Design review of the part built by this model. Coordinates are the model's own, in mm. Face numbers are marked on the shaded views. A direction names the side the tool comes from. Give positions to 0.01 mm unless a question says otherwise; leave off trailing zeros. Write each loop counter-clockwise with the first axis right and the second up, starting at its lowest first coordinate (ties: lowest second). Pieces come first, ordered by that corner, then holes. Notation, with made-up numbers: (48.5, 23.5) -> (81.5, 23.5) arc R13 ccw to (81.5, 33.5) -> close; hole circle Ø11 at (74.5, 84.25). An arc over 180 degrees is marked (long way). Put each result on its own line as item: value. Start each with the question number.
Solid Edge part; units mm, degrees
sketch "Sketch1" plane through (0, 0, 0) normal (0, -1, 0) x (1, 0, 0)
  line L0 (0, 27.23) -> (27.065, 27.23)
  line L1 (27.065, 27.23) -> (27.065, 11.95)
  line L2 (19.9, 11.95) -> (27.065, 11.95)
  line L3 (19.9, 10.05) -> (19.9, 11.95)
  line L4 (18.87, 10.05) -> (19.9, 10.05)
  line L5 (18.87, 8.05) -> (18.87, 10.05)
  line L6 (7.4, 8.05) -> (18.87, 8.05)
  line L7 (7.4, 8.05) -> (3.6, 0)
  line L8 (2, 0) -> (3.6, 0)
  line L9 (2, 0) -> (2, 8.38)
  line L10 (2, 8.38) -> (0, 8.38)
  line L11 (0, 8.38) -> (0, 27.23)
revolve "RevolvedProtrusion1" add sketch "Sketch1" angle 360 about axis through (0, 0, 8.38) along (0, 0, 1)
sketch "Sketch2" plane through (0, 0, 0) normal (1, 0, 0) x (0, 1, 0)
  circle A0 centre (0, 15.9202) radius 3
extrude "ExtrudedProtrusion_2" add sketch "Sketch2" along normal blind 42.065 and the other way blind 3.3012
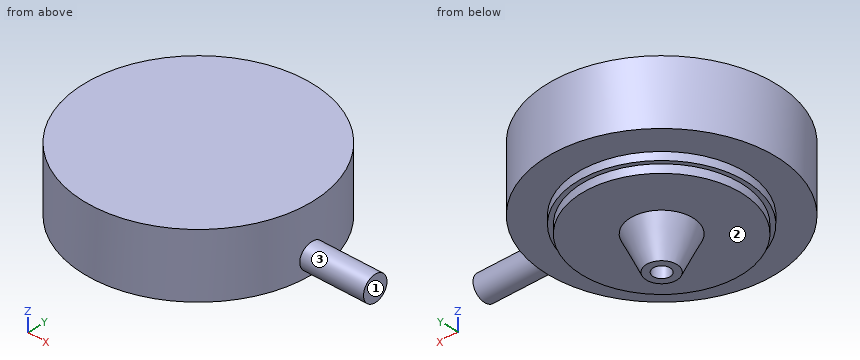
Q1. To check wall thickness, follow probe 1 along Z at (x, y) = (-19, -4); probe 2 along Z at (x, y) = (5, -9); probe 3 along Y at (x, z) = (0, 3.5). State the ranges of each line that lie inside material, in increasing order. Write a range as from..to.
Q2. Take a section at C-C on z = 20.75. Give the boundary of the cut face in (x, y) (3 decimals), then the cut area to 3 significant figures.
Q3. Take a section at A-A on y = 0. Give the boundary of the cut face in (x, z) (3 decimals), then the cut area to 3 significant figures.
Q4. Take a section at B-B on x = 0. Give the boundary of the cut face in (y, z) (3 decimals).
Q5. Take a section at D-D on x = -12. Give the boundary of the cut face in (y, z), then the cut area to 3 significant figures.
Q6. For pin 1 (6 mm diameter, centred on x = -9.5, z = 14, fed in from -Y); pin 2 (3 mm diameter, centred on x = 5.5, y = 21.5, fed in from -Z); pin 3 (1.5 mm diameter, centred on y = -17, z = 6.5, fed in from +X); pin 4 (1 mm diameter, centred on y = -3.5, z = 8.5, fed in from +X), all flat-tipped, find the tip position at first contact; note any pin that passes through.
Q7. Machinability: for the marked faces 1, 2 and 3, which of the approach directions +Z, -Z, +X, -X, +Y, -Y give a long, thin tool a straight path to every point of the face, cutting with its end or side? Answer none if there is none.
Result:
1. probe 1: z = 10.05..27.23
1. probe 2: z = 8.05..27.23
1. probe 3: y = -5.25..-2, 2..5.25
2. outline: circle Ø54.13 at (0, 0)
2. area: 2,300 mm^2
3. outline: (-27.065, 11.95) -> (-19.9, 11.95) -> (-19.9, 10.05) -> (-18.87, 10.05) -> (-18.87, 8.05) -> (-7.4, 8.05) -> (-3.6, 0) -> (-2, 0) -> (-2, 8.38) -> (2, 8.38) -> (2, 0) -> (3.6, 0) -> (7.4, 8.05) -> (18.87, 8.05) -> (18.87, 10.05) -> (19.9, 10.05) -> (19.9, 11.95) -> (27.065, 11.95) -> (27.065, 12.92) -> (42.065, 12.92) -> (42.065, 18.92) -> (27.065, 18.92) -> (27.065, 27.23) -> (-27.065, 27.23) -> close
3. area: 1,120 mm^2
4. outline: (-27.065, 11.95) -> (-19.9, 11.95) -> (-19.9, 10.05) -> (-18.87, 10.05) -> (-18.87, 8.05) -> (-7.4, 8.05) -> (-3.6, 0) -> (-2, 0) -> (-2, 8.38) -> (2, 8.38) -> (2, 0) -> (3.6, 0) -> (7.4, 8.05) -> (18.87, 8.05) -> (18.87, 10.05) -> (19.9, 10.05) -> (19.9, 11.95) -> (27.065, 11.95) -> (27.065, 27.23) -> (-27.065, 27.23) -> close
5. outline: (-24.26, 11.95) -> (-15.87, 11.95) -> (-15.87, 10.05) -> (-14.56, 10.05) -> (-14.56, 8.05) -> (14.56, 8.05) -> (14.56, 10.05) -> (15.87, 10.05) -> (15.87, 11.95) -> (24.26, 11.95) -> (24.26, 27.23) -> (-24.26, 27.23) -> close
5. area: 860 mm^2
6. pin 1: stops at y = -26.27
6. pin 2: stops at z = 11.95
6. pin 3: passes through
6. pin 4: stops at x = 18.63
7. face 1: +Z, -Z, +X, +Y, -Y
7. face 2: -Z
7. face 3: +X
